The listing builds one solid part. Answer for the finished solid, in the listing's coordinates (mm). Face numbers are marked on the shaded views. Round coordinates to 2 decimals unless told otherwise and drop trailing zeros. Order: outer loops, then holes, each group sorted by start corner. A loop starts at its lowest first (then second) coordinate and runs counter-clockwise, first axis right, second up. Notation, with made-up numbers: M 51,69 L 55,69 A16 ccw 55,85 Z; hole C 56.5,22 d10. An arc over 180 degrees is marked long. Write item = value, one per line. Start each with the question number.
(1) A cutting plane is placed at A-A, the plane x = -57. Determine the outline of the cut face in (y, z), and give its area (3 significant figures).
(2) For a pull along X with two mould halves and no side action, classify the marked faces 1 and 2 as released by +X, released by -X, zero draft, split by the parting line, or undercut.
(3) A cutting plane is placed at C-C, the plane y = 126.5. Determine the outline of the cut face in (x, z).
(4) Each of these flat-tipped pins is pushed along its axis until it touches: pin 1 (0.6 mm diameter, centred on y = 1049.5, z = -8, fed in from +X); pin 2 (10 mm diameter, centred on x = -81, z = -13.5, fed in from -Y); pin 3 (2 mm diameter, centred on y = 826.5, z = 13, fed in from -X); pin 4 (1.1 mm diameter, centred on x = -94.5, z = -0.5, fed in from -Y). Where does it stop, or does it pass through?
(5) A cutting plane is placed at B-B, the plane y = 579. Determine the outline of the cut face in (x, z).
(6) Straight lines are drawn through the part: probe 1 along X at (y, z) = (667.5, 12); probe 2 along X at (y, z) = (711.5, -18.5); probe 3 along Z at (x, y) = (-73, 697). For each, find the intervals that lie inside material, in ascending order. Write a range as from..to.
from build123d import *

# Parameters (mm, degrees)
BASE_FLANGE1_DEPTH             = 1050
CUT_EXTRUDE1_REACH             = 1056.479
EDGE_FLANGE5_STRIP_W           = 16
EDGE_FLANGE5_STRIP_H           = 1
EDGE_FLANGE5_STRIP_CUT_DEPTH   = 54
EDGE_FLANGE5_STRIP_2_W         = 16
EDGE_FLANGE5_STRIP_2_H         = 1
EDGE_FLANGE5_STRIP_CUT_2_DEPTH = 14
EDGE_FLANGE5_DEPTH             = 54
EDGE_FLANGE5_BEND_DEPTH        = 14
EDGE_FLANGE7_DEPTH             = 1048
EDGE_FLANGE8_STRIP_W           = 6
EDGE_FLANGE8_STRIP_H           = 1
EDGE_FLANGE8_STRIP_CUT_DEPTH   = 16
EDGE_FLANGE8_DEPTH             = 16
EDGE_FLANGE9_START             = 529.5
EDGE_FLANGE9_DEPTH             = 515.5
EDGE_FLANGE9_2_DEPTH           = 0.5
EDGE_FLANGE9_START_2           = 530
EDGE_FLANGE9_3_DEPTH           = 515


# Read off the part's stored shape, not the designer's step: Edge-Flange9
# Sheet-metal steps are written as plain solids
with BuildPart() as part:
    # Sketch1 → Base-Flange1 (new body)
    with BuildSketch(Plane(origin=(0, 0, 0), x_dir=(1, 0, 0), z_dir=(0, 1, 0))):
        with BuildLine():
            Line((0, 0), (-14, 0))
            ThreePointArc((-14, 0), (-14.707106781, -0.292893219), (-15, -1))
            Line((-15, -1), (-15, -18))
            ThreePointArc((-15, -18), (-15.585786438, -19.414213562), (-17, -20))
            Line((-17, -20), (-33, -20))
            ThreePointArc((-33, -20), (-34.414213562, -19.414213562), (-35, -18))
            Line((-35, -18), (-35, -1))
            ThreePointArc((-35, -1), (-35.292893219, -0.292893219), (-36, 0))
            Line((-36, 0), (-95, 0))
            Line((-95, 0), (-95, 1))
            Line((-95, 1), (-36, 1))
            ThreePointArc((-36, 1), (-34.585786438, 0.414213562), (-34, -1))
            Line((-34, -1), (-34, -18))
            ThreePointArc((-34, -18), (-33.707106781, -18.707106781), (-33, -19))
            Line((-33, -19), (-17, -19))
            ThreePointArc((-17, -19), (-16.292893219, -18.707106781), (-16, -18))
            Line((-16, -18), (-16, -1))
            ThreePointArc((-16, -1), (-15.414213562, 0.414213562), (-14, 1))
            Line((-14, 1), (0, 1))
            Line((0, 1), (0, 0))
        make_face()
    extrude(amount=BASE_FLANGE1_DEPTH)

    # Sketch18 → Cut-Extrude1 (cut, up to next)
    with BuildSketch(Plane.XY, mode=Mode.PRIVATE) as cut_extrude1_sk1:
        with BuildLine():
            Line((-95, 1045), (-95, 1050))
            Line((-95, 1050), (-90, 1050))
            ThreePointArc((-90, 1050), (-93.535533906, 1048.535533906), (-95, 1045))
        make_face()
    cut_extrude1_tool1 = extrude(cut_extrude1_sk1.sketch, amount=-CUT_EXTRUDE1_REACH, mode=Mode.PRIVATE) & part.part
    add(cut_extrude1_tool1.solids().sort_by_distance((-93.88316, 1048.88316, 0))[0], mode=Mode.SUBTRACT)

    # Edge-Flange5 strip (across the edge) → Edge-Flange5 strip cut (cut)
    with BuildSketch(Plane(origin=(-90, 1050, -1), x_dir=(0, -1, 0), z_dir=(1, 0, 0))):
        with Locations((-6, -0.5)):
            Rectangle(EDGE_FLANGE5_STRIP_W, EDGE_FLANGE5_STRIP_H)
    extrude(amount=EDGE_FLANGE5_STRIP_CUT_DEPTH, mode=Mode.SUBTRACT)

    # Edge-Flange5 strip 2 (across the edge) → Edge-Flange5 strip cut 2 (cut)
    with BuildSketch(Plane(origin=(-14, 1050, -1), x_dir=(0, -1, 0), z_dir=(1, 0, 0))):
        with Locations((-6, -0.5)):
            Rectangle(EDGE_FLANGE5_STRIP_2_W, EDGE_FLANGE5_STRIP_2_H)
    extrude(amount=EDGE_FLANGE5_STRIP_CUT_2_DEPTH, mode=Mode.SUBTRACT)

    # Edge-Flange5 section (across the edge) → Edge-Flange5 (add)
    with BuildSketch(Plane(origin=(-90, 1050, -1), x_dir=(0, -1, 0), z_dir=(1, 0, 0))):
        with BuildLine():
            Line((0, 1), (0, 19))
            Line((0, 19), (1, 19))
            Line((1, 19), (1, 1))
            ThreePointArc((1, 1), (1.292893219, 0.292893219), (2, 0))
            Line((2, 0), (2, -1))
            ThreePointArc((2, -1), (0.585786438, -0.414213562), (0, 1))
        make_face()
    extrude(amount=EDGE_FLANGE5_DEPTH)

    # Edge-Flange5 section 2 (across the edge) → Edge-Flange5 bend (add)
    with BuildSketch(Plane(origin=(-14, 1050, -1), x_dir=(0, -1, 0), z_dir=(1, 0, 0))):
        with BuildLine():
            Line((0, 1), (0, 19))
            Line((0, 19), (1, 19))
            Line((1, 19), (1, 1))
            ThreePointArc((1, 1), (1.292893219, 0.292893219), (2, 0))
            Line((2, 0), (2, -1))
            ThreePointArc((2, -1), (0.585786438, -0.414213562), (0, 1))
        make_face()
    extrude(amount=EDGE_FLANGE5_BEND_DEPTH)

    # Edge-Flange7 section (across the edge) → Edge-Flange7 (add)
    with BuildSketch(Plane(origin=(1, 1048, -1), x_dir=(-1, 0, 0), z_dir=(0, -1, 0))):
        with BuildLine():
            Line((-1, 1), (-1, 29))
            Line((-1, 29), (0, 29))
            Line((0, 29), (0, 1))
            ThreePointArc((0, 1), (0.292893219, 0.292893219), (1, 0))
            Line((1, 0), (1, -1))
            ThreePointArc((1, -1), (-0.414213562, -0.414213562), (-1, 1))
        make_face()
    extrude(amount=EDGE_FLANGE7_DEPTH)

    # Edge-Flange8 strip (across the edge) → Edge-Flange8 strip cut (cut)
    with BuildSketch(Plane(origin=(-33, 1050, 19), x_dir=(0, -1, 0), z_dir=(1, 0, 0))):
        with Locations((-1, -0.5)):
            Rectangle(EDGE_FLANGE8_STRIP_W, EDGE_FLANGE8_STRIP_H)
    extrude(amount=EDGE_FLANGE8_STRIP_CUT_DEPTH, mode=Mode.SUBTRACT)

    # Edge-Flange8 section (across the edge) → Edge-Flange8 (add)
    with BuildSketch(Plane(origin=(-33, 1050, 19), x_dir=(0, -1, 0), z_dir=(1, 0, 0))):
        with BuildLine():
            Line((0, 1), (0, 29))
            Line((0, 29), (1, 29))
            Line((1, 29), (1, 1))
            ThreePointArc((1, 1), (1.292893219, 0.292893219), (2, 0))
            Line((2, 0), (2, -1))
            ThreePointArc((2, -1), (0.585786438, -0.414213562), (0, 1))
        make_face()
    extrude(amount=EDGE_FLANGE8_DEPTH)

    # Edge-Flange9 outline → Edge-Flange9 (cut)
    with BuildSketch(Plane(origin=(0, 0, 0), x_dir=(1, 0, 0), z_dir=(0, 1, 0)).offset(EDGE_FLANGE9_START)):
        with BuildLine():
            ThreePointArc((-93, 0), (-94, 0.267949193), (-94.732050807, 1))
            Line((-94.732050807, 1), (-95, 1))
            Line((-95, 1), (-95, 0))
            Line((-95, 0), (-93, 0))
        make_face()
    extrude(amount=EDGE_FLANGE9_DEPTH, mode=Mode.SUBTRACT)

    # Edge-Flange9 2 outline → Edge-Flange9 2 (cut)
    with BuildSketch(Plane(origin=(0, 0, 0), x_dir=(1, 0, 0), z_dir=(0, 1, 0)).offset(EDGE_FLANGE9_START)):
        with BuildLine():
            Line((-92.5, 1), (-94.732050807, 1))
            ThreePointArc((-94.732050807, 1), (-94, 0.267949193), (-93, 0))
            Line((-93, 0), (-92.5, 0))
            Line((-92.5, 0), (-92.5, 1))
        make_face()
    extrude(amount=EDGE_FLANGE9_2_DEPTH, mode=Mode.SUBTRACT)

    # Edge-Flange9 3 outline → Edge-Flange9 3 (add)
    with BuildSketch(Plane(origin=(0, 0, 0), x_dir=(1, 0, 0), z_dir=(0, 1, 0)).offset(EDGE_FLANGE9_START_2)):
        with BuildLine():
            Line((-95, 21), (-95, 2))
            ThreePointArc((-95, 2), (-94.931851652, 1.48236191), (-94.732050807, 1))
            Line((-94.732050807, 1), (-93, 1))
            ThreePointArc((-93, 1), (-93.707106781, 1.292893219), (-94, 2))
            Line((-94, 2), (-94, 21))
            Line((-94, 21), (-95, 21))
        make_face()
    extrude(amount=EDGE_FLANGE9_3_DEPTH)


solid = part.part
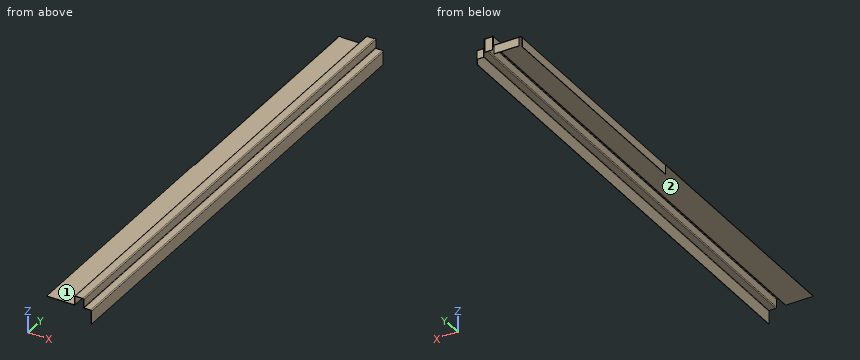
Reported:
q1.outline = M 0,-1 L 1048,-1 A1 cw 1049,-2 L 1049,-20 L 1050,-20 L 1050,-2 A2 ccw 1048,0 L 0,0 Z
q1.area = 1,070 mm²
q2.face_1 = zero draft
q2.face_2 = undercut
q3.outline = M -95,-1 L -36,-1 A2 ccw -34,1 L -34,18 A1 cw -33,19 L -17,19 A1 cw -16,18 L -16,1 A2 ccw -14,-1 L 0,-1 A1 cw 1,-2 L 1,-30 L 2,-30 L 2,-2 A2 ccw 0,0 L -14,0 A1 cw -15,1 L -15,18 A2 ccw -17,20 L -33,20 A2 ccw -35,18 L -35,1 A1 cw -36,0 L -95,0 Z
q4.pin_1 = 0
q4.pin_2 = 1049
q4.pin_3 = -35
q4.pin_4 = 0
q5.outline = M -95,-21 L -94,-21 L -94,-2 A1 cw -93,-1 L -36,-1 A2 ccw -34,1 L -34,18 A1 cw -33,19 L -17,19 A1 cw -16,18 L -16,1 A2 ccw -14,-1 L 0,-1 A1 cw 1,-2 L 1,-30 L 2,-30 L 2,-2 A2 ccw 0,0 L -14,0 A1 cw -15,1 L -15,18 A2 ccw -17,20 L -33,20 A2 ccw -35,18 L -35,1 A1 cw -36,0 L -93,0 A2 ccw -95,-2 Z
q6.probe_1 = -35..-34, -16..-15
q6.probe_2 = -95..-94, 1..2
q6.probe_3 = -1..0
